Design review of the part built by this model. Coordinates are the model's own, in mm. A direction names the side the tool comes from. Coordinates: 2 decimals unless noted, no trailing zeros. Order: outer loops, then holes, each group sorted by start corner. A loop starts at its lowest first (then second) coordinate and runs counter-clockwise, first axis right, second up. Notation, with made-up numbers: (0, 25.5) -> (34, 25.5) arc R36 cw to (34, 61.5) -> close; hole circle Ø8 at (41, 79.5). An arc over 180 degrees is marked (long way). Write item = value, one per line.
Autodesk Inventor part; units mm, degrees
ref_plane "YZ Plane" through (0, 0, 0) normal (1, 0, 0) x (0, 1, 0)
ref_plane "XZ Plane" through (0, 0, 0) normal (0, 1, 0) x (-1, 0, 0)
ref_plane "XY Plane" through (0, 0, 0) normal (0, 0, 1) x (1, 0, 0)
sketch "Sketch1" plane through (0, 0, 0) normal (0, 1, 0) x (-1, 0, 0)
  line L0 (9.5, 13.75) -> (-9.5, 13.75)
  line L1 (-9.5, 13.75) -> (-9.5, -13.75)
  line L2 (-9.5, -13.75) -> (9.5, -13.75)
  line L3 (9.5, -13.75) -> (9.5, 13.75)
  point P0 (0, 0)
  dimension "d0" = 19
  dimension "d1" = 27.5
  dimension "d2" = 13.75
  dimension "d3" = 9.5
extrude "Extrusion1" add sketch "Sketch1" along normal blind 27
sketch "Sketch2" plane through (0, 27, 0) normal (0, 1, 0) x (1, 0, 0)
  line L0 (9.5, 13.75) -> (-9.5, 13.75)
  line L1 (9.5, -13.75) -> (9.5, 13.75)
  line L2 (-9.5, -13.75) -> (9.5, -13.75)
  line L3 (-9.5, 13.75) -> (-9.5, -13.75)
  line L4 (-6.5, -12.75) -> (6.5, -12.75)
  line L5 (6.5, -12.75) -> (6.5, 12.75)
  line L6 (6.5, 12.75) -> (-6.5, 12.75)
  line L7 (-6.5, 12.75) -> (-6.5, -12.75)
  point P0 (0, 0)
  dimension "d6" = 3
  dimension "d7" = 3
  dimension "d8" = 1
  dimension "d9" = 1
extrude "Extrusion2" cut sketch "Sketch2" against normal blind 24 contours L7 L6 L5 L4
sketch "Sketch3" plane through (-9.5, 0, 13.75) normal (0, 0, 1) x (1, 0, 0)
  line L0 (0, 27) -> (19, 27)
  line L1 (3, 27) -> (3, 3)
  line L2 (16, 27) -> (16, 3)
  line L3 (3, 27) -> (3, 3)
  line L4 (16, 27) -> (16, 3)
  line L5 (3, 27) -> (16, 27)
  line L6 (16, 27) -> (16, 23)
  line L7 (16, 23) -> (3, 23)
  line L8 (3, 23) -> (3, 27)
  point P0 (9.5, 0)
  point P1 (3, 23)
  dimension "d12" = 4
extrude "Extrusion3" cut sketch "Sketch3" against normal blind 30
fillet "Fillet1" radius 3 4 edges at (-8, 27, 13.75) (-8, 27, -13.75) (8, 27, -13.75) (8, 27, 13.75)
sketch "Sketch4" plane through (0, 0, 0) normal (0, -1, 0) x (1, 0, 0)
  circle A0 centre (0, 0) radius 2
  circle A1 centre (0, -9) radius 2
  circle A2 centre (0, 9) radius 2
  dimension "d16" = 4
  dimension "d17" = 4
  dimension "d18" = 4
  dimension "d19" = 9
  dimension "d20" = 9
extrude "Extrusion4" cut sketch "Sketch4" against normal blind 5
sketch "Sketch5" plane through (9.5, 0, 13.75) normal (1, 0, 0) x (0, 0, -1)
  line L0 (3, 27) -> (24.5, 27)
  line L1 (27.5, 0) -> (27.5, 24)
  line L2 (0, 0) -> (0, 24)
  circle A0 centre (13.75, 13) radius 2
  circle A1 centre (22.25, 13) radius 2
  circle A2 centre (5.25, 13) radius 2
  line L3 (1.7351, 17.75) -> (24.75, 17.75) construction
  circle A3 centre (13.75, 22.5) radius 2
  circle A4 centre (22.25, 22.5) radius 2
  circle A5 centre (5.25, 22.5) radius 2
  point P0 (13.75, 0)
  dimension "d23" = 14
  dimension "d24" = 27.5
  dimension "d25" = 13.75
  dimension "d26" = 4
  dimension "d27" = 0
  dimension "d28" = 0
  dimension "d29" = 4
  dimension "d30" = 4
  dimension "d31" = 8.5
  dimension "d32" = 8.5
  dimension "d35" = 4.75
hole "Hole1" at (9.5, 22.5, 8.5) at (9.5, 22.5, 0) at (9.5, 22.5, -8.5) at (9.5, 13, 0) at (9.5, 13, -8.5) at (9.5, 13, 8.5) direction (-1, 0, 0) diameter 4 end through all
sketch "Sketch6" plane through (-6.5, 3, 12.75) normal (1, 0, 0) x (0, 0, -1)
  circle A0 centre (12.75, 10) radius 2
  line L0 (6.75, 16) -> (18.75, 16)
  line L1 (18.75, 16) -> (18.75, 4)
  line L2 (18.75, 4) -> (6.75, 4)
  line L3 (6.75, 4) -> (6.75, 16)
  point P0 (12.75, -3)
  dimension "d43" = 12
  dimension "d44" = 12
  dimension "d45" = 6
  dimension "d46" = 6
extrude "Extrusion5" add sketch "Sketch6" along normal blind 1
sketch "Sketch7" plane through (6.5, 3, -12.75) normal (-1, 0, 0) x (0, 0, 1)
  line L0 (6.75, 16) -> (18.75, 16)
  line L1 (6.75, 4) -> (6.75, 16)
  line L2 (18.75, 16) -> (18.75, 4)
  line L3 (18.75, 4) -> (6.75, 4)
  circle A0 centre (12.75, 10) radius 2
  line L4 (18.75, 16) -> (6.75, 16)
  line L5 (6.75, 16) -> (6.75, 4)
  line L6 (6.75, 4) -> (18.75, 4)
  line L7 (18.75, 4) -> (18.75, 16)
  point P0 (12.75, -3)
extrude "Extrusion6" add sketch "Sketch7" along normal blind 1
sketch "Sketch8" plane through (-9.5, 0, -13.75) normal (-1, 0, 0) x (0, 0, 1)
  circle A0 centre (13.75, 13) radius 2
  circle A1 centre (13.75, 13) radius 5
  point P0 (13.75, 0)
  dimension "d51" = 10
extrude "Extrusion7" cut sketch "Sketch8" against normal through all
equation "\"d16\" = d17"
equation "\"d18\" = d17"
equation "\"d25\" = 0.5 * d24"
equation "\"d29\" = d26"
equation "\"d30\" = d26"
properties part number "SoporteEncoder" material "Plastic, Opaque Black"
(1) We need section B-B (x = -0.75). Write out the cut boundary in (y, z), and give its area (3 significant figures).
Report:
outline = (0, -13.75) -> (23, -13.75) -> (23, -12.75) -> (3, -12.75) -> (3, -10.85) -> (0, -10.85) -> close; (0, -7.15) -> (3, -7.15) -> (3, -1.85) -> (0, -1.85) -> close; (0, 1.85) -> (3, 1.85) -> (3, 7.15) -> (0, 7.15) -> close; (0, 10.85) -> (3, 10.85) -> (3, 12.75) -> (23, 12.75) -> (23, 13.75) -> (0, 13.75) -> close
area = 89.1 mm²
(2) The part is to be moulded in two halves that separate along Y. For faces 1 (the cylindrical face through (-7.98, 26.14, 12.85)), 2 (the flat face through (6, 13, 6)), 3 (the cylindrical face through (-8.021, 20.517, 8.76)), say which applies: released by +Y, released by -Y, zero draft, split by the parting line, or undercut.
Report:
face_1 = released by +Y
face_2 = zero draft
face_3 = undercut
(3) We need section C-C (z = 9). Write out the cut boundary in (x, y), and give its area (3 significant figures).
Report:
outline = (-9.5, 0) -> (-2, 0) -> (-2, 3) -> (-6.5, 3) -> (-6.5, 11.06) -> (-9.5, 11.06) -> close; (-9.5, 14.94) -> (-6.5, 14.94) -> (-6.5, 20.56) -> (-9.5, 20.56) -> close; (-9.5, 24.44) -> (-6.5, 24.44) -> (-6.5, 27) -> (-9.5, 27) -> close; (2, 0) -> (9.5, 0) -> (9.5, 11.06) -> (6.5, 11.06) -> (6.5, 3) -> (2, 3) -> close; (6.5, 14.94) -> (9.5, 14.94) -> (9.5, 20.56) -> (6.5, 20.56) -> close; (6.5, 24.44) -> (9.5, 24.44) -> (9.5, 27) -> (6.5, 27) -> close
area = 143 mm²
(4) We need section D-D (y = 22.5). Give the number of separate pieces and of enclosed holes in the cut face, and give its area (3 significant figures).
Report:
separate_pieces = 6
enclosed_holes = 0
area = 119 mm²
(5) For faces 4 (the flat face through (6, 7, 0)), 5 (the flat face through (0, 23, 13)), 6 (the flat face through (6, 13, -6)), list the 3-axis set-ups (+Z, -Z, +X, -X, +Y, -Y) from which the entire face can be reached by the end or side of a thin tool; tool diameter is ignored.
Report:
face_4 = none
face_5 = +Z, -Z, +Y
face_6 = +Y
(6) Insertion check: pin 1 (10 mm diameter, centred on x = 3.5, z = 11, fed in from -Y); pin 2 (2.5 mm diameter, centred on y = 13, z = 8.5, fed in from +X); pin 3 (4 mm diameter, centred on x = 1.5, z = -9.5, fed in from +Y). Each pin has a flat end and moves straight along its axis. Give the tip position at first contact, or say it passes through.
Report:
pin_1 = 0
pin_2 = through
pin_3 = 3
(7) We need section A-A (y = 17). Write out the cut boundary in (x, z).
Report:
outline = (-9.5, -13.75) -> (9.5, -13.75) -> (9.5, -3) -> (5.5, -3) -> (5.5, -6) -> (6.5, -6) -> (6.5, -12.75) -> (-6.5, -12.75) -> (-6.5, -6) -> (-5.5, -6) -> (-5.5, -3) -> (-9.5, -3) -> close; (-9.5, 3) -> (-5.5, 3) -> (-5.5, 6) -> (-6.5, 6) -> (-6.5, 12.75) -> (6.5, 12.75) -> (6.5, 6) -> (5.5, 6) -> (5.5, 3) -> (9.5, 3) -> (9.5, 13.75) -> (-9.5, 13.75) -> close
(8) For L1, parallel to Z at x = -8.6, y = 22.5; L2, parallel to Z at x = 0, y = 2.15; L3, parallel to Y at x = 7.9, z = -8.5, list the stretches that pass through material, from the lowest coordinate up.
Report:
L1 = -13.75 to -10.5, -6.5 to -2, 2 to 6.5, 10.5 to 13.75
L2 = -13.75 to -11, -7 to -2, 2 to 7, 11 to 13.75
L3 = 0 to 11, 15 to 20.5, 24.5 to 27
